```python
from build123d import *

# Parameters (mm, degrees)
ESQUISSE1_R             = 1.5
BOSS_EXTRU_1_DEPTH      = 3
ESQUISSE2_R             = 1.25
ENL_V_MAT_EXTRU_2_DEPTH = 10


with BuildPart() as part:
    # Esquisse1 → Boss.-Extru.1 (new body)
    with BuildSketch(Plane.XY):
        with BuildLine():
            Line((-26.749397242, -0.17957503), (-24.145347662, -22.5))
            Line((-24.145347662, -22.5), (24.145347662, -22.5))
            Line((24.145347662, -22.5), (26.749397242, -0.17957503))
            ThreePointArc((26.749397242, -0.17957503), (0, 26.75), (-26.749397242, -0.17957503))
        make_face()
        with Locations((0, -19.45)):
            Circle(ESQUISSE1_R, mode=Mode.SUBTRACT)
        with Locations((-16.844194104, 9.725)):
            Circle(ESQUISSE1_R, mode=Mode.SUBTRACT)
        with Locations((16.844194104, 9.725)):
            Circle(ESQUISSE1_R, mode=Mode.SUBTRACT)
    extrude(amount=BOSS_EXTRU_1_DEPTH)

    # Esquisse2 → Enlèv. mat.-Extru.2 (cut)
    with BuildSketch(Plane.XY.offset(3)):
        with Locations((21.029790949, -19.001295206)):
            Circle(ESQUISSE2_R)
        with Locations((13.354846659, 19.031830461)):
            Circle(ESQUISSE2_R)
        with Locations((-13.354846659, 19.031830461)):
            Circle(ESQUISSE2_R)
        with Locations((-21.029790949, -19.001295206)):
            Circle(ESQUISSE2_R)
    extrude(amount=-ENL_V_MAT_EXTRU_2_DEPTH, mode=Mode.SUBTRACT)


solid = part.part
```
Verification items for the finished model (mm, model axes). Coordinates: 2 decimals unless noted, no trailing zeros. Write each loop counter-clockwise with the first axis right and the second up, starting at its lowest first coordinate (ties: lowest second). Pieces come first, ordered by that corner, then holes. Notation, with made-up numbers: M -26,-29 L 18,-29 A4 ccw 18,-24 Z; hole C 28.25,-33.75 d1. An arc over 180 degrees is marked long. Answer as a JSON object with one key per item and string values. Group by question number.
(1) Cross-section at C-C, the plane x = 17. Record the cut outline in (y, z), and give its area (3 significant figures).
(2) Release check for a two-part mould opening along X. For faces 1 (the face through (0.591, 26.743, 1.479)), 2 (the face through (-14.276, 19.877, 1.521)), 3 (the face through (25.43, -11.5, 1.48)), 4 (the face through (0, 2, 0)) record: +X half, -X half, draft (parallel to the pull), parting line (faces both ways), or undercut.
(3) Cross-section at B-B, the plane z = 1.15. Record the cut outline in (x, y) (3 decimals), and give its area (3 significant figures).
(4) Gauge pin test, flat end, axial feed: pin 1 (1.5 mm diameter, centred on x = 13.35, y = 19.03, fed in from +Z). Record the tip position at first contact, or that the pin passes through.
(5) Material ranges on line 1 (X direction, y = 11.5, z = 2.7); line 2 (X direction, y = 10, z = 1.9); line 3 (Y direction, x = 20, z = 0.2), recorded low to high.
(6) Cross-section at D-D, the plane y = -16. Record the cut outline in (x, z), and give its area (3 significant figures).
(7) Cross-section at A-A, the plane x = 0. Record the cut outline in (y, z).
Reply:
{
 "1": {"outline": "M -22.5,0 L 8.23,0 L 8.23,3 L -22.5,3 Z; M 11.22,0 L 20.65,0 L 20.65,3 L 11.22,3 Z", "area": "121 mm²"},
 "2": {"face 1": "parting line", "face 2": "undercut", "face 3": "+X half", "face 4": "draft"},
 "3": {"outline": "M -26.749,-0.18 L -24.145,-22.5 L 24.145,-22.5 L 26.749,-0.18 A26.75 ccw long Z; hole C -21.03,-19.001 d2.5; hole C -16.844,9.725 d3; hole C -13.355,19.032 d2.5; hole C 0,-19.45 d3; hole C 13.355,19.032 d2.5; hole C 16.844,9.725 d3; hole C 21.03,-19.001 d2.5", "area": "2,230 mm²"},
 "4": {"pin 1": "through"},
 "5": {"line 1": "-24.15 to 24.15", "line 2": "-24.81 to -18.32, -15.37 to 15.37, 18.32 to 24.81", "line 3": "-22.5 to -19.71, -18.29 to 17.76"},
 "6": {"outline": "M -24.9,0 L 24.9,0 L 24.9,3 L -24.9,3 Z", "area": "149 mm²"},
 "7": {"outline": "M -22.5,0 L -20.95,0 L -20.95,3 L -22.5,3 Z; M -17.95,0 L 26.75,0 L 26.75,3 L -17.95,3 Z"}
}
